CAD build for the part. Positions are in the model's coordinates, mm. Round coordinates to 2 decimals unless told otherwise and drop trailing zeros. Order: outer loops, then holes, each group sorted by start corner. A loop starts at its lowest first (then second) coordinate and runs counter-clockwise, first axis right, second up. Notation, with made-up numbers: M -35.75,20 L 6.25,20 A7 cw 6.25,24 Z; hole C 38,81.5 d4. An arc over 180 degrees is marked long. Answer as a JSON object with one key per item and string values. Group by question number.
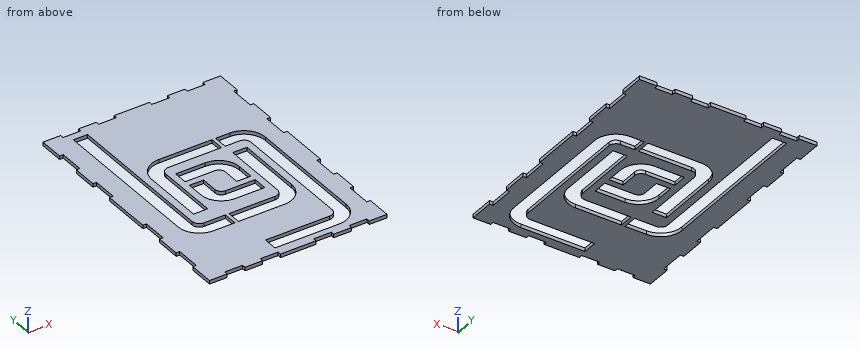
```python
from build123d import *

# Parameters (mm, degrees)
F1_DEPTH = 5


with BuildPart() as f1:
    # F0 (on Top) → F1 (new body)
    with BuildSketch(Plane.XY):
        Polygon((38.337818, -187.449847), (43.337818, -187.449847), (43.337818, -182.449847), (43.337818, -152.449847), (38.337818, -152.449847), (38.337818, -117.449847), (43.337818, -117.449847), (43.337818, -82.449847), (38.337818, -82.449847), (38.337818, -47.449847), (43.337818, -47.449847), (43.337818, 22.550153), (38.337818, 22.550153), (38.337818, 57.550153), (43.337818, 57.550153), (43.337818, 92.550153), (38.337818, 92.550153), (38.337818, 127.550153), (43.337818, 127.550153), (43.337818, 157.550153), (43.337818, 162.550153), (18.337818, 162.550153), (18.337818, 157.550153), (-6.662182, 157.550153), (-6.662182, 162.550153), (-31.662182, 162.550153), (-31.662182, 157.550153), (-56.662182, 157.550153), (-56.662182, 162.550153), (-81.662182, 162.550153), (-106.662182, 162.550153), (-106.662182, 157.550153), (-131.662182, 157.550153), (-131.662182, 162.550153), (-156.662182, 162.550153), (-156.662182, 157.550153), (-181.662182, 157.550153), (-181.662182, 162.550153), (-206.662182, 162.550153), (-206.662182, 127.550153), (-201.662182, 127.550153), (-201.662182, 92.550153), (-206.662182, 92.550153), (-206.662182, 57.550153), (-201.662182, 57.550153), (-201.662182, 22.550153), (-206.662182, 22.550153), (-206.662182, -12.449847), (-206.662182, -47.449847), (-201.662182, -47.449847), (-201.662182, -82.449847), (-206.662182, -82.449847), (-206.662182, -117.449847), (-201.662182, -117.449847), (-201.662182, -152.449847), (-206.662182, -152.449847), (-206.662182, -187.449847), (-201.662182, -187.449847), (-181.662182, -187.449847), (-181.662182, -182.449847), (-156.662182, -182.449847), (-156.662182, -187.449847), (-131.662182, -187.449847), (-131.662182, -182.449847), (-106.662182, -182.449847), (-106.662182, -187.449847), (-81.662182, -187.449847), (-56.662182, -187.449847), (-56.662182, -182.449847), (-31.662182, -182.449847), (-31.662182, -187.449847), (-6.662182, -187.449847), (-6.662182, -182.449847), (18.337818, -182.449847), (18.337818, -187.449847), align=None)
        with BuildLine():
            Line((-4.479525, -143.196979), (-4.479525, 26.803021))
            ThreePointArc((-4.479525, 26.803021), (-7.408457, 33.874089), (-14.479525, 36.803021))
            Line((-14.479525, 36.803021), (-34.410654, 36.803021))
            Line((-34.410654, 36.803021), (-34.410654, 56.803021))
            Line((-34.410654, 56.803021), (-14.479525, 56.803021))
            ThreePointArc((-14.479525, 56.803021), (6.733678, 48.016224), (15.520475, 26.803021))
            Line((15.520475, 26.803021), (15.520475, -143.196979))
            ThreePointArc((15.520475, -143.196979), (6.733678, -164.410183), (-14.479525, -173.196979))
            Line((-14.479525, -173.196979), (-104.812019, -173.196979))
            Line((-104.812019, -173.196979), (-104.812019, -153.196979))
            Line((-104.812019, -153.196979), (-14.479525, -153.196979))
            ThreePointArc((-14.479525, -153.196979), (-7.408457, -150.268047), (-4.479525, -143.196979))
        make_face(mode=Mode.SUBTRACT)
        with BuildLine():
            Line((-94.812019, -8.145639), (-94.812019, -32.145639))
            ThreePointArc((-94.812019, -32.145639), (-92.191017, -38.473298), (-85.863359, -41.0943))
            Line((-85.863359, -41.0943), (-44.198371, -41.0943))
            Line((-44.198371, -41.0943), (-44.198371, -61.0943))
            Line((-44.198371, -61.0943), (-85.863359, -61.0943))
            ThreePointArc((-85.863359, -61.0943), (-106.333153, -52.615433), (-114.812019, -32.145639))
            Line((-114.812019, -32.145639), (-114.812019, -8.145639))
            Line((-114.812019, -8.145639), (-94.812019, -8.145639))
        make_face(mode=Mode.SUBTRACT)
        with BuildLine():
            Line((-109.385459, -83.196979), (-44.479525, -83.196979))
            ThreePointArc((-44.479525, -83.196979), (-37.408457, -80.268047), (-34.479525, -73.196979))
            Line((-34.479525, -73.196979), (-34.479525, 20.803021))
            Line((-34.479525, 20.803021), (-14.479525, 20.803021))
            Line((-14.479525, 20.803021), (-14.479525, -73.196979))
            ThreePointArc((-14.479525, -73.196979), (-23.266322, -94.410183), (-44.479525, -103.196979))
            Line((-44.479525, -103.196979), (-109.385459, -103.196979))
            Line((-109.385459, -103.196979), (-109.385459, -83.196979))
        make_face(mode=Mode.SUBTRACT)
        with BuildLine():
            Line((-154.479525, 146.803021), (-154.479525, -73.196979))
            ThreePointArc((-154.479525, -73.196979), (-151.550593, -80.268047), (-144.479525, -83.196979))
            Line((-144.479525, -83.196979), (-114.385459, -83.196979))
            Line((-114.385459, -83.196979), (-114.385459, -103.196979))
            Line((-114.385459, -103.196979), (-144.479525, -103.196979))
            ThreePointArc((-144.479525, -103.196979), (-165.692728, -94.410183), (-174.479525, -73.196979))
            Line((-174.479525, -73.196979), (-174.479525, 146.803021))
            Line((-174.479525, 146.803021), (-154.479525, 146.803021))
        make_face(mode=Mode.SUBTRACT)
        with BuildLine():
            Line((-39.410654, 36.803021), (-114.479525, 36.803021))
            ThreePointArc((-114.479525, 36.803021), (-121.550593, 33.874089), (-124.479525, 26.803021))
            Line((-124.479525, 26.803021), (-124.479525, -61.0943))
            Line((-124.479525, -61.0943), (-144.479525, -61.0943))
            Line((-144.479525, -61.0943), (-144.479525, 26.803021))
            ThreePointArc((-144.479525, 26.803021), (-135.692728, 48.016224), (-114.479525, 56.803021))
            Line((-114.479525, 56.803021), (-39.410654, 56.803021))
            Line((-39.410654, 56.803021), (-39.410654, 36.803021))
        make_face(mode=Mode.SUBTRACT)
        with BuildLine():
            Line((-44.198371, -32.145639), (-64.198371, -32.145639))
            Line((-64.198371, -32.145639), (-64.198371, -8.145639))
            ThreePointArc((-64.198371, -8.145639), (-66.819373, -1.817981), (-73.147031, 0.803021))
            Line((-73.147031, 0.803021), (-114.812019, 0.803021))
            Line((-114.812019, 0.803021), (-114.812019, 20.803021))
            Line((-114.812019, 20.803021), (-73.147031, 20.803021))
            ThreePointArc((-73.147031, 20.803021), (-52.677237, 12.324154), (-44.198371, -8.145639))
            Line((-44.198371, -8.145639), (-44.198371, -32.145639))
        make_face(mode=Mode.SUBTRACT)
    extrude(amount=F1_DEPTH)


solid = f1.part
```
Item 1: Drill centre lines: line 1 (Y direction, x = -77.5, z = 0.55); line 2 (Y direction, x = -31, z = 0.5); line 3 (X direction, y = 38.5, z = 1). Where is each one in solid material? Low to high. Write a range as [from, to].
Item 2: Cut at C-C, the plane y = 133. Give the cut face in (x, z), and give its area (3 significant figures).
Item 3: Cut at D-D, the plane y = -13. Give the cut face in (x, z), and give its area (3 significant figures).
Item 4: Cut at A-A, the plane y = -69.5. Give the cut face in (x, z).
Item 5: Flat gauge pins, fed straight in: pin 1 Ø2.5 at (y, z) = (-53.5, 3.5) entering from -X; pin 2 Ø10 at (x, y) = (-161.5, 12.5) entering from +Z; pin 3 Ø1.5 at (x, z) = (-167.5, 3.5) entering from -Y. Where does each tip first touch, or does it go through?
Item 6: Cut at B-B, the plane x = 2.5. Give the cut face in (y, z).
Response values:
{
 "1": {"line 1": "[-187.45, -173.2], [-153.2, -103.2], [-83.2, -61.09], [-41.09, 0.8], [20.8, 36.8], [56.8, 162.55]", "line 2": "[-187.45, -173.2], [-153.2, -100], [20.8, 36.8], [56.8, 162.55]", "line 3": "[-201.66, -174.48], [-154.48, -142.11], [-39.41, -34.41], [13.15, 38.34]"},
 "2": {"outline": "M -206.66,0 L -174.48,0 L -174.48,5 L -206.66,5 Z; M -154.48,0 L 43.34,0 L 43.34,5 L -154.48,5 Z", "area": "1,150 mm^2"},
 "3": {"outline": "M -206.66,0 L -174.48,0 L -174.48,5 L -206.66,5 Z; M -154.48,0 L -144.48,0 L -144.48,5 L -154.48,5 Z; M -124.48,0 L -114.81,0 L -114.81,5 L -124.48,5 Z; M -94.81,0 L -64.2,0 L -64.2,5 L -94.81,5 Z; M -44.2,0 L -34.48,0 L -34.48,5 L -44.2,5 Z; M -14.48,0 L -4.48,0 L -4.48,5 L -14.48,5 Z; M 15.52,0 L 43.34,0 L 43.34,5 L 15.52,5 Z", "area": "650 mm^2"},
 "4": {"outline": "M -201.66,0 L -174.48,0 L -174.48,5 L -201.66,5 Z; M -154.48,0 L -34.48,0 L -34.48,5 L -154.48,5 Z; M -14.48,0 L -4.48,0 L -4.48,5 L -14.48,5 Z; M 15.52,0 L 38.34,0 L 38.34,5 L 15.52,5 Z"},
 "5": {"pin 1": "x = -201.66", "pin 2": "through", "pin 3": "y = -182.45"},
 "6": {"outline": "M -182.45,0 L -167.93,0 L -167.93,5 L -182.45,5 Z; M 51.54,0 L 157.55,0 L 157.55,5 L 51.54,5 Z"}
}
